from build123d import *

# Parameters (mm, degrees)
SKETCH_1_R                   = 35.5
SKETCH_1_R_2                 = 2.75
EXTRUDE_1_DEPTH              = 9
SKETCH_2_R                   = 4.5
CUT_EXTRUDE_1_DEPTH          = 5.5
EXTRUDE_2_DEPTH              = 11.5
FILLET_1_R                   = 4
EXTRUDE_3_DEPTH              = 18.5
HOLE_WIZARD_M5_1_D           = 4.2
HOLE_WIZARD_M5_1_DEPTH       = 7.5
HOLE_WIZARD_M5_1_TIP         = 1.2618073
CUT_EXTRUDE_3_DEPTH          = 64.572792923
CUT_EXTRUDE_3_DEPTH_BACK     = 64.572792923
SKETCH_13_R                  = 2.85
SKETCH_14_R                  = 5
CUT_EXTRUDE_4_DEPTH          = 87.846128416
SKETCH_15_R                  = 5
CUT_EXTRUDE_5_DEPTH          = 87.846128416
HOLE_WIZARD_2_5_2_5_1_REACH  = 56.229
HOLE_WIZARD_2_5_2_5_1_BORE_R = 1.25
SKETCH_19_R                  = 12.5
CUT_EXTRUDE_6_DEPTH          = 7
CUT_EXTRUDE_6_DRAFT          = -15
SKETCH_20_R                  = 15.5
CUT_EXTRUDE_7_DEPTH          = 9
FILLET_2_R                   = 2


with BuildPart() as part:
    # 스케치1 → 보스-돌출1 (new body)
    with BuildSketch(Plane(origin=(0, 0, 0), x_dir=(1, 0, 0), z_dir=(0, 1, 0))):
        with Locations(Location((0, 0, 0), (0, 0, 270))):
            Circle(SKETCH_1_R)
        with Locations(Location((0, 29.5, 0), (0, 0, 270))):
            Circle(SKETCH_1_R_2, mode=Mode.SUBTRACT)
        with Locations(Location((25.547749412, 14.75, 0), (0, 0, 270))):
            Circle(SKETCH_1_R_2, mode=Mode.SUBTRACT)
        with Locations(Location((25.547749412, -14.75, 0), (0, 0, 270))):
            Circle(SKETCH_1_R_2, mode=Mode.SUBTRACT)
        with Locations(Location((0, -29.5, 0), (0, 0, 270))):
            Circle(SKETCH_1_R_2, mode=Mode.SUBTRACT)
        with Locations(Location((-25.547749412, -14.75, 0), (0, 0, 270))):
            Circle(SKETCH_1_R_2, mode=Mode.SUBTRACT)
        with Locations(Location((-25.547749412, 14.75, 0), (0, 0, 270))):
            Circle(SKETCH_1_R_2, mode=Mode.SUBTRACT)
    extrude(amount=EXTRUDE_1_DEPTH)

    # 스케치2 → 컷-돌출1 (cut)
    with BuildSketch(Plane(origin=(0, 9, 0), x_dir=(1, 0, 0), z_dir=(0, 1, 0))):
        with Locations(Location((0, 29.5, 0), (0, 0, 270))):
            Circle(SKETCH_2_R)
        with Locations(Location((25.548249412, 14.750866025, 0), (0, 0, 270))):
            Circle(SKETCH_2_R)
        with Locations(Location((25.549249412, -14.749133975, 0), (0, 0, 270))):
            Circle(SKETCH_2_R)
        with Locations(Location((0.002, -29.5, 0), (0, 0, 270))):
            Circle(SKETCH_2_R)
        with Locations(Location((-25.546249412, -14.750866025, 0), (0, 0, 270))):
            Circle(SKETCH_2_R)
        with Locations(Location((-25.547249412, 14.749133975, 0), (0, 0, 270))):
            Circle(SKETCH_2_R)
    extrude(amount=-CUT_EXTRUDE_1_DEPTH, mode=Mode.SUBTRACT)

    # 스케치3 → 보스-돌출2 (add)
    with BuildSketch(Plane(origin=(0, 9, 0), x_dir=(1, 0, 0), z_dir=(0, 1, 0))):
        with BuildLine():
            ThreePointArc((35.5, 0), (35.299107366, 3.771341825), (34.698703146, 7.5))
            Line((34.698703146, 7.5), (22.534695472, 7.5))
            ThreePointArc((22.534695472, 7.5), (0, 23.75), (-22.534695472, 7.5))
            Line((-22.534695472, 7.5), (-34.698703146, 7.5))
            ThreePointArc((-34.698703146, 7.5), (-35.5, 0), (-34.698703146, -7.5))
            Line((-34.698703146, -7.5), (-22.534695472, -7.5))
            ThreePointArc((-22.534695472, -7.5), (0, -23.75), (22.534695472, -7.5))
            Line((22.534695472, -7.5), (34.698703146, -7.5))
            ThreePointArc((34.698703146, -7.5), (35.299107366, -3.771341825), (35.5, 0))
        make_face()
    extrude(amount=EXTRUDE_2_DEPTH)

    # 필렛1
    fillet_1_edges = [part.edges().sort_by_distance(p)[0] for p in [
        (22.534695472, 14.75, -7.5),
        (-22.534695472, 14.75, -7.5),
        (-22.534695472, 14.75, 7.5),
        (22.534695472, 14.75, 7.5),
    ]]
    fillet(fillet_1_edges, radius=FILLET_1_R)

    # 스케치8 → 보스-돌출3 (add)
    with BuildSketch(Plane(origin=(0, 20.5, 0), x_dir=(1, 0, 0), z_dir=(0, 1, 0))):
        with BuildLine():
            Line((-4.513584937, 20.642857143), (-12.720103003, 8.857142857))
            ThreePointArc((-12.720103003, 8.857142857), (-15.5, 0), (-12.720103003, -8.857142857))
            Line((-12.720103003, -8.857142857), (-4.513584937, -20.642857143))
            ThreePointArc((-4.513584937, -20.642857143), (0, -23), (4.513584937, -20.642857143))
            Line((4.513584937, -20.642857143), (12.720103003, -8.857142857))
            ThreePointArc((12.720103003, -8.857142857), (15.5, 0), (12.720103003, 8.857142857))
            Line((12.720103003, 8.857142857), (4.513584937, 20.642857143))
            ThreePointArc((4.513584937, 20.642857143), (0, 23), (-4.513584937, 20.642857143))
        make_face()
    extrude(amount=EXTRUDE_3_DEPTH)

    # M5 나사 구멍1
    with Locations(Plane(origin=(0, 39, 0), x_dir=(1, 0, 0), z_dir=(0, 1, 0))):
        with Locations((0, 17.5), (0, -17.5)):
            Hole(HOLE_WIZARD_M5_1_D / 2, depth=HOLE_WIZARD_M5_1_DEPTH)
            with Locations((0, 0, -(HOLE_WIZARD_M5_1_DEPTH + HOLE_WIZARD_M5_1_TIP / 2))):  # 118° drill point
                Cone(0, HOLE_WIZARD_M5_1_D / 2, HOLE_WIZARD_M5_1_TIP, mode=Mode.SUBTRACT)

    # 스케치13 → 컷-돌출3 (cut, two sides: drawn at the far end of the back side and taken through both)
    with BuildSketch(Plane(origin=(0, 0, 0), x_dir=(0, 0, -1), z_dir=(1, 0, 0)).offset(-CUT_EXTRUDE_3_DEPTH_BACK)):
        with Locations((0, 9)):
            Circle(SKETCH_13_R)
    extrude(amount=CUT_EXTRUDE_3_DEPTH + CUT_EXTRUDE_3_DEPTH_BACK, mode=Mode.SUBTRACT)

    # 스케치14 → 컷-돌출4 (cut, through all)
    with BuildSketch(Plane(origin=(33.5, 0, 0), x_dir=(0, 0, -1), z_dir=(1, 0, 0))):
        with Locations(Location((0, 9, 0), (0, 0, 270))):
            Circle(SKETCH_14_R)
    extrude(amount=CUT_EXTRUDE_4_DEPTH, mode=Mode.SUBTRACT)

    # 스케치15 → 컷-돌출5 (cut, through all)
    with BuildSketch(Plane(origin=(-33.5, 0, 0), x_dir=(0, 0, -1), z_dir=(1, 0, 0))):
        with Locations(Location((0, 9, 0), (0, 0, 270))):
            Circle(SKETCH_15_R)
    extrude(amount=-CUT_EXTRUDE_5_DEPTH, mode=Mode.SUBTRACT)

    # Ø2.5 (2.5) 지름 구멍1 bore → Ø2.5 (2.5) 지름 구멍1 (cut, up to next)
    with BuildSketch(Plane(origin=(0, 20.5, 0), x_dir=(1, 0, 0), z_dir=(0, 1, 0)), mode=Mode.PRIVATE) as hole_wizard_2_5_2_5_1_sk1:
        with Locations((23, 0)):
            Circle(HOLE_WIZARD_2_5_2_5_1_BORE_R)
    hole_wizard_2_5_2_5_1_tool1 = extrude(hole_wizard_2_5_2_5_1_sk1.sketch, amount=-HOLE_WIZARD_2_5_2_5_1_REACH, mode=Mode.PRIVATE) & part.part
    # Ø2.5 (2.5) 지름 구멍1 bore → Ø2.5 (2.5) 지름 구멍1 (cut, up to next)
    with BuildSketch(Plane(origin=(0, 20.5, 0), x_dir=(1, 0, 0), z_dir=(0, 1, 0)), mode=Mode.PRIVATE) as hole_wizard_2_5_2_5_1_sk2:
        with Locations((-23, 0)):
            Circle(HOLE_WIZARD_2_5_2_5_1_BORE_R)
    hole_wizard_2_5_2_5_1_tool2 = extrude(hole_wizard_2_5_2_5_1_sk2.sketch, amount=-HOLE_WIZARD_2_5_2_5_1_REACH, mode=Mode.PRIVATE) & part.part
    add(hole_wizard_2_5_2_5_1_tool1.solids().sort_by_distance((23, 20.5, 0))[0], mode=Mode.SUBTRACT)
    add(hole_wizard_2_5_2_5_1_tool2.solids().sort_by_distance((-23, 20.5, 0))[0], mode=Mode.SUBTRACT)

    # 스케치10 → 컷-회전1 (revolve, cut)
    with BuildSketch(Plane.XY, mode=Mode.PRIVATE) as cut_revolve_1_sk:
        Polygon((11.5, 39), (11.5, 20.5), (7.5, 20.5), (7.5, 0), (0, 0), (0, 39), align=None)
    revolve(cut_revolve_1_sk.sketch.rotate(Axis((0, 0, 0), (0, 1, 0)), 90), axis=Axis((0, 0, 0), (0, 1, 0)), mode=Mode.SUBTRACT)


with BuildPart() as cut_extrude_6_tool:
    # 스케치19 → 컷-돌출6 (with draft: the straight prism first)
    with BuildSketch(Plane(origin=(0, 9, 0), x_dir=(-1, 0, 0), z_dir=(0, -1, 0))):
        Circle(SKETCH_19_R)
    extrude(amount=-CUT_EXTRUDE_6_DEPTH)
    # 컷-돌출6: the draft: its side faces are tilted about the plane it starts from
    cut_extrude_6_sides = [cut_extrude_6_tool.faces().sort_by_distance(p)[0] for p in [
        (12.5, 12.5, 0),
    ]]
    draft(cut_extrude_6_sides, Plane(origin=(0, 9, 0), x_dir=(-1, 0, 0), z_dir=(0, -1, 0)), CUT_EXTRUDE_6_DRAFT)


with BuildPart() as part_1:
    add(part.part)

    # 컷-돌출6: cut by cut_extrude_6_tool
    add(cut_extrude_6_tool.part, mode=Mode.SUBTRACT)

    # 스케치20 → 컷-돌출7 (cut)
    with BuildSketch(Plane.XZ):
        with Locations(Location((0, 0, 0), (0, 0, 270))):
            Circle(SKETCH_20_R)
    extrude(amount=-CUT_EXTRUDE_7_DEPTH, mode=Mode.SUBTRACT)

    # 필렛2
    fillet_2_edges = [part_1.edges().sort_by_distance(p)[0] for p in [
        (10.624355653, 16, 0),
    ]]
    fillet(fillet_2_edges, radius=FILLET_2_R)


solid = part_1.part
Build history of the part. All positions in model axes, mm. A direction names the side the tool comes from. Round coordinates to 2 decimals unless told otherwise and drop trailing zeros. Loops run counter-clockwise (first coordinate to the right, second up) from the corner with the lowest first, then second, coordinate; pieces in that order, holes last. Notation, with made-up numbers: (56, 87.25) -> (70, 87.25) arc R14 cw to (70, 105.25) -> close; hole circle Ø6 at (1, -28.75). An arc over 180 degrees is marked (long way). Use CSV: the item, a comma, the result in double quotes. Start each with the question number.
Q1. Flat gauge pins, fed straight in: pin 1 Ø6 at (x, y) = (16.5, 10.5) entering from -Z; pin 2 Ø4.5 at (x, y) = (30, 15) entering from +Z; pin 3 Ø2 at (y, z) = (5.5, 17.5) entering from -X. Where does each tip first touch, or does it go through?
Q2. Mould opens along X. For faces 1 (the face through (-25.427, 1.726, 12.003)), 2 (the face through (15.5, 29.6, 0.1)), 3 (the face through (0, 9, 24)) say: +X half, -X half, draft (parallel to the pull), parting line (faces both ways), or undercut.
Q3. Which spindle directions (+Z, -Z, +X, -X, +Y, -Y) get a long thin tool onto all of the face, cutting with end or side? Do faces 4 (the face through (-30, 15, -7.5)), 5 (the face through (23.064, 14.83, 8.154)), 6 (the face through (8, 20.5, 0)), 7 (the face through (2.1, 16, -7.4)). Say none if no direction does.
Q4. Saw through at B-B on z = 29.5. Give the cut face in (x, y).
Q5. Saw through at A-A on z = -30.5. Give the cut face in (x, y).
Q6. Drill centre lines: L1, parallel to Z at x = 0, y = 2.4; L2, parallel to Y at x = 28, z = 0; L3, parallel to X at y = 30, z = 0. Where is each one in solid material? Low to high.
Solutions:
1,pin 1,"stops at z = -32.66"
1,pin 2,"stops at z = 7.5"
1,pin 3,"stops at x = -31.43"
2,face 1,"undercut"
2,face 2,"+X half"
2,face 3,"draft"
3,face 4,"-Z, -X, +Y"
3,face 5,"+Z, +X, +Y"
3,face 6,"+Y"
3,face 7,"-Y"
4,outline,"(-19.75, 0) -> (-2.75, 0) -> (-2.75, 3.5) -> (-4.5, 3.5) -> (-4.5, 9) -> (-19.75, 9) -> close; (2.75, 0) -> (19.75, 0) -> (19.75, 9) -> (4.5, 9) -> (4.5, 3.5) -> (2.75, 3.5) -> close"
5,outline,"(-18.17, 0) -> (-2.56, 0) -> (-2.56, 3.5) -> (-4.39, 3.5) -> (-4.39, 9) -> (-18.17, 9) -> close; (2.56, 0) -> (18.17, 0) -> (18.17, 9) -> (4.39, 9) -> (4.39, 3.5) -> (2.56, 3.5) -> close"
6,L1,"z = -35.5 to -32.25, -26.75 to -15.5, 15.5 to 26.75, 32.25 to 35.5"
6,L2,"y = 0 to 6.15, 11.85 to 20.5"
6,L3,"x = -15.5 to -11.5, 11.5 to 15.5"
